```python
from build123d import *

# Parameters (mm, degrees)
MODEL_R             = 1.449999899
MODEL_R_2           = 1.450000076
BOSS_EXTRUDE1_DEPTH = 5.85


with BuildPart() as part:
    # Model → Boss-Extrude1 (new body)
    with BuildSketch(Plane.XY):
        with BuildLine():
            Line((508.267115634, 556.488649767), (505.831367634, 543.517354767))
            ThreePointArc((505.831367634, 543.517354767), (506.791253617, 539.812058859), (510.255750143, 538.184833401))
            Line((510.255750143, 538.184833401), (529.708723634, 538.184833401))
            ThreePointArc((529.708723634, 538.184833401), (533.173220159, 539.812058859), (534.133106143, 543.517354767))
            Line((534.133106143, 543.517354767), (531.697358143, 556.488649767))
            Line((531.697358143, 556.488649767), (531.697358143, 578.551691787))
            ThreePointArc((531.697358143, 578.551691787), (530.236877746, 582.07760337), (526.710966163, 583.538083767))
            Line((526.710966163, 583.538083767), (524.199056888, 583.538083767))
            Line((524.199056888, 583.538083767), (524.199056888, 577.792158))
            Line((524.199056888, 577.792158), (525.982236888, 577.762664))
            Line((525.982236888, 577.762664), (525.982236888, 555.093173))
            Line((525.982236888, 555.093173), (513.982236888, 555.093173))
            Line((513.982236888, 555.093173), (513.982236888, 577.762664))
            Line((513.982236888, 577.762664), (515.765416888, 577.792158))
            Line((515.765416888, 577.792158), (515.765416888, 583.538083767))
            Line((515.765416888, 583.538083767), (513.253507613, 583.538083767))
            ThreePointArc((513.253507613, 583.538083767), (509.727596031, 582.07760337), (508.267115634, 578.551691787))
            Line((508.267115634, 578.551691787), (508.267115634, 556.488649767))
        make_face()
        with Locations(Location((509.982236888, 542.200965, 0), (0, 0, 180))):
            Circle(MODEL_R, mode=Mode.SUBTRACT)
        with Locations((519.982236888, 542.200965)):
            Circle(MODEL_R_2, mode=Mode.SUBTRACT)
        with Locations((529.982236888, 542.200965)):
            Circle(MODEL_R, mode=Mode.SUBTRACT)
    extrude(amount=BOSS_EXTRUDE1_DEPTH)


solid = part.part
```
Could you check a few things on this model? Use its own coordinates, in mm. A direction names the side the tool comes from. Round coordinates to 2 decimals unless told otherwise and drop trailing zeros. Write each loop counter-clockwise with the first axis right and the second up, starting at its lowest first coordinate (ties: lowest second). Pieces come first, ordered by that corner, then holes.
(1) Suppose I cut it at A-A on y = 570.5. Write out the boundary of the cut face in (x, z).
Findings below:
outline: (508.27, 0) - (513.98, 0) - (513.98, 5.85) - (508.27, 5.85) - close; (525.98, 0) - (531.7, 0) - (531.7, 5.85) - (525.98, 5.85) - close
(2) Suppose I cut it at D-D on y = 554.5. Write out the boundary of the cut face in (x, z), and give its area (3 significant figures).
Findings below:
outline: (507.89, 0) - (532.07, 0) - (532.07, 5.85) - (507.89, 5.85) - close
area: 141 mm2
(3) Which directions (+Z, -Z, +X, -X, +Y, -Y) give clear straight access to the entire face, cutting with the end or side of a thin tool? Please do faces 4 (the face through (520, 555.093, 3)), 5 (the face through (520, 538.185, 3)), 6 (the face through (508.267, 568, 3)).
Findings below:
face 4: +Z, -Z
face 5: +Z, -Z, +X, -X, -Y
face 6: +Z, -Z, -X, +Y
(4) Suppose I cut it at B-B on x = 525. Write out the boundary of the cut face in (y, z).
Findings below:
outline: (538.18, 0) - (555.09, 0) - (555.09, 5.85) - (538.18, 5.85) - close; (577.78, 0) - (583.54, 0) - (583.54, 5.85) - (577.78, 5.85) - close
(5) Thinking about a two-plate mould opening in X: for faces 1 (the face through (531.697, 567, 3)), 2 (the face through (525, 583.538, 3)), 3 (the face through (524.199, 581, 3)), which applies, +X half, -X half, draft (parallel to the pull), parting line (faces both ways), or undercut?
Findings below:
face 1: +X half
face 2: draft
face 3: undercut
(6) If I drill on probe 1 along X at (y, z) = (559.5, 2.9); probe 2 along X at (y, z) = (543, 5.3); probe 3 along X at (y, z) = (543.5, 4.35), over which ranges is the centre line in solid material (lowest first)?
Findings below:
probe 1: x = 508.27 to 513.98, 525.98 to 531.7
probe 2: x = 505.76 to 508.77, 511.19 to 518.77, 521.19 to 528.77, 531.19 to 534.2
probe 3: x = 505.83 to 509.34, 510.63 to 519.34, 520.63 to 529.34, 530.63 to 534.14
(7) For pin 1 (1.7 mm diameter, centred on y = 581.5, z = 3, fed in from +X); pin 2 (1.7 mm diameter, centred on y = 582, z = 2, fed in from -X); pin 3 (2 mm diameter, centred on y = 567.5, z = 1.5, fed in from -X); pin 4 (2.5 mm diameter, centred on x = 509.98, y = 542.2, fed in from -Z), each with a flat end and sliding along its axis, tell me the tip position at first contact or that it passes through.
Findings below:
pin 1: stops at x = 531.23
pin 2: stops at x = 509
pin 3: stops at x = 508.27
pin 4: passes through
(8) Suppose I cut it at C-C on z = 3.2. Write out the boundary of the cut face in (x, y), and give its area (3 significant figures).
Findings below:
outline: (505.83, 543.52) arc R4.5 ccw to (510.26, 538.18) - (529.71, 538.18) arc R4.5 ccw to (534.13, 543.52) - (531.7, 556.49) - (531.7, 578.55) arc R4.99 ccw to (526.71, 583.54) - (524.2, 583.54) - (524.2, 577.79) - (525.98, 577.76) - (525.98, 555.09) - (513.98, 555.09) - (513.98, 577.76) - (515.77, 577.79) - (515.77, 583.54) - (513.25, 583.54) arc R4.99 ccw to (508.27, 578.55) - (508.27, 556.49) - close; hole circle Ø2.9 at (509.98, 542.2); hole circle Ø2.9 at (519.98, 542.2); hole circle Ø2.9 at (529.98, 542.2)
area: 761 mm2
